For this review, use the dimensioned drawing (mm, ordinates from the lowest corner) and the shaded views. Round coordinates to 2 decimals unless told otherwise and drop trailing zeros. Loops run counter-clockwise (first coordinate to the right, second up) from the corner with the lowest first, then second, coordinate; pieces in that order, holes last. Notation, with made-up numbers: M 19,-7.5 L 47,-7.5 A17 cw 47,14.5 Z; hole C 12.5,-2.5 d2. An arc over 180 degrees is marked long. Use a Markdown table: item, result. Add a question column.
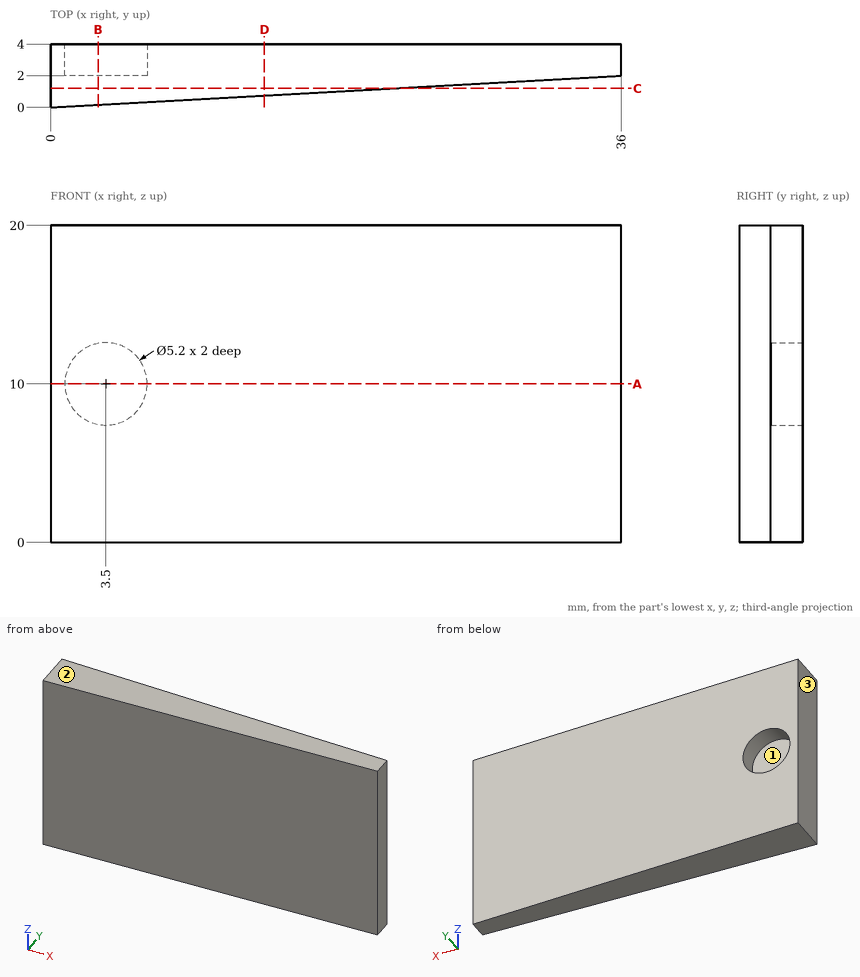
(1) Insertion check: pin 1 Ø4 at (x, z) = (26, 17.5) entering from -Y; pin 2 Ø5 at (x, z) = (22, 6.5) entering from -Y. Each pin has a flat end and moves straight along its axis. Give the tip position at first contact, or say it passes through.
(2) To check wall thickness, follow probe 1 along X at (y, z) = (3.5, 10); probe 2 along Z at (x, y) = (3.5, 3); probe 3 along Y at (x, z) = (22, 19.25). State the ranges of each line that lie inside material, in increasing order.
(3) Consider section C-C, the plane y = 1.2. Give the boundary of the cut face in (x, z), then the cut area to 3 significant figures.
(4) Consider section D-D, the plane x = 13.5. Give the boundary of the cut face in (y, z).
(5) Consider section B-B, the plane x = 3. Give the boundary of the cut face in (y, z).
(6) Consider section A-A, the plane z = 10. Give the boundary of the cut face in (x, y).
(7) Draft analysis for pull direction Z (two halves, no side actions). For the marked faces 1, 2 and 3, state which applies: released by +Z, released by -Z, zero draft, split by the parting line, or undercut.
Found:
| question | item | result |
|---|---|---|
| 1 | pin 1 | stops at y = 1.33 |
| 1 | pin 2 | stops at y = 1.08 |
| 2 | probe 1 | x = 0 to 0.9, 6.1 to 36 |
| 2 | probe 2 | z = 0 to 7.4, 12.6 to 20 |
| 2 | probe 3 | y = 1.22 to 4 |
| 3 | outline | M 0,0 L 21.6,0 L 21.6,20 L 0,20 Z |
| 3 | area | 432 mm^2 |
| 4 | outline | M 0.75,0 L 4,0 L 4,20 L 0.75,20 Z |
| 5 | outline | M 0.17,0 L 4,0 L 4,7.45 L 2,7.45 L 2,12.55 L 4,12.55 L 4,20 L 0.17,20 Z |
| 6 | outline | M 0,0 L 36,2 L 36,4 L 6.1,4 L 6.1,2 L 0.9,2 L 0.9,4 L 0,4 Z |
| 7 | face 1 | undercut |
| 7 | face 2 | released by +Z |
| 7 | face 3 | zero draft |
